from build123d import *

# Parameters (mm, degrees)
PAD_DEPTH       = 90
POCKET_DEPTH    = 8.9110010593
POCKET001_DEPTH = 7.0820946587


with BuildPart() as part:
    # Sketch → Pad (new body)
    with BuildSketch(Plane.YZ):
        with BuildLine():
            Line((-7, -25), (-4, -25))
            ThreePointArc((-4, -25), (-3.2928932188, -24.7071067812), (-3, -24))
            Line((-3, -24), (-3, 0))
            ThreePointArc((3, 0), (0, 1), (-3, 0))
            Line((3, 0), (3, -4))
            ThreePointArc((3, -4), (3.2928932188, -4.7071067812), (4, -5))
            Line((5.124826301, -5), (4, -5))
            ThreePointArc((5.124826301, -5), (5.6328573812, -4.8613387379), (6, -4.483808843))
            Line((14.00686173, 10), (6, -4.483808843))
            Line((14.00686173, 10), (14.00686173, 11.5))
            ThreePointArc((14.00686173, 11.5), (13.7139685112, 12.2071067812), (13.00686173, 12.5))
            Line((13.00686173, 12.5), (10.00686173, 12.5))
            ThreePointArc((10.00686173, 12.5), (9.2997549488, 12.2071067812), (9.00686173, 11.5))
            Line((9.00686173, 11.5), (9.00686173, 10))
            ThreePointArc((-2.99313827, 10), (3.00686173, 6.7888974491), (9.00686173, 10))
            Line((-2.99313827, 10), (-5.0865765197, 49.9451813902))
            ThreePointArc((-5.0865765197, 49.9451813902), (-5.4160754481, 50.6359902594), (-6.1375420107, 50.8914749687))
            Line((-6.1375420107, 50.8914749687), (-9.133430615, 50.7344671))
            ThreePointArc((-9.133430615, 50.7344671), (-9.8242394842, 50.4049681716), (-10.0797241935, 49.683501609))
            Line((-10.0797241935, 49.683501609), (-8, 10))
            Line((-8, 10), (-8, -24))
            ThreePointArc((-8, -24), (-7.7071067812, -24.7071067812), (-7, -25))
        make_face()
    extrude(amount=PAD_DEPTH)

    # Sketch002 (on Face1 of Pad) → Pocket (cut, through all)
    with BuildSketch(Plane(origin=(0, -2.4622975914, -0.1290435487), x_dir=(0, -0.0523359562, 0.9986295348), z_dir=(0, 0.9986295348, 0.0523359562))):
        with BuildLine():
            Line((51.1429441011, 75), (45.1429441011, 75))
            ThreePointArc((45.1429441011, 75), (15.1429441011, 45), (45.1429441011, 15))
            Line((45.1429441011, 15), (51.1429441011, 15))
            Line((51.1429441011, 15), (51.1429441011, 75))
        make_face()
    extrude(amount=-POCKET_DEPTH, mode=Mode.SUBTRACT)

    # Sketch003 (on Face17 of Pocket) → Pocket001 (cut, through all)
    with BuildSketch(Plane.ZX.offset(-3)):
        with BuildLine():
            Line((-75, 75), (-35, 75))
            ThreePointArc((-35, 15), (-5, 45), (-35, 75))
            Line((-35, 15), (-75, 15))
            Line((-75, 15), (-75, 75))
        make_face()
    extrude(amount=-POCKET001_DEPTH, mode=Mode.SUBTRACT)


solid = part.part
The listing builds one solid part. Answer for the finished solid, in the listing's coordinates (mm). A direction names the side the tool comes from. Round coordinates to 2 decimals unless told otherwise and drop trailing zeros. Order: outer loops, then holes, each group sorted by start corner. A loop starts at its lowest first (then second) coordinate and runs counter-clockwise, first axis right, second up. Notation, with made-up numbers: (73.5, -19) -> (106.5, -19) arc R14 ccw to (106.5, -8) -> close; hole circle Ø11 at (-18, -27). An arc over 180 degrees is marked (long way). Write each question's results on one line, items separated by ' | '. Start each with the question number.
Q1. Which of the six approach directions +Z, -Z, +X, -X, +Y, -Y give full straight-line access (tool end or side, diameter ignored) to faces 1 (the flat face through (44, 12, 12.5)), 2 (the flat face through (15, -7, 48)), 3 (the flat face through (44, -3, -4)), 4 (the flat face through (90, -3.4, 10.3))?
Q2. The mould has two halves that part along Y. Classify faces 5 (the flat face through (44, 3, -2)), 6 (the flat face through (44, -8, -3)), 7 (the flat face through (75, -7, 48)): pulls with the +Y half, pulls with the -Y half, needs draft (parallel to the pull), parting line crosses it, or undercut.
Q3. Find section A-A (x = 9). Determine the outline of the cut face in (y, z).
Q4. Find section D-D (x = 50). Determine the outline of the cut face in (y, z), then the cut area to 3 significant figures.
Q5. Find section B-B (z = -8). Determine the outline of the cut face in (x, y).
Q6. Find section C-C (y = 7.75). Determine the outline of the cut face in (x, z).
Q7. Each of these flat-tipped pins is pushed along its axis until it touches: pin 1 (1 mm diameter, centred on x = 68.5, y = 1, fed in from -Z); pin 2 (12 mm diameter, centred on x = 20.5, z = 7.5, fed in from -Y); pin 3 (1.2 mm diameter, centred on x = 43.5, z = 11, fed in from -Y). Where does it stop, or does it pass through?
Q8. Straight lines are drawn through the part: probe 1 along Y at (x, z) = (4.5, -18); probe 2 along Y at (x, z) = (36, -4.5); probe 3 along Y at (x, z) = (81, 47.5). For each, find the intervals that lie inside material, in ascending order. Write a range as from..to.
Worked answers:
1) face 1: +Z, +X, -X, +Y | face 2: +Z, +Y, -Y | face 3: -Z, +X, -X | face 4: +Z, -Z, +X, +Y, -Y
2) face 5: undercut | face 6: pulls with the -Y half | face 7: needs draft
3) outline: (-10.08, 49.68) -> (-8, 10) -> (-8, -24) arc R1 ccw to (-7, -25) -> (-4, -25) arc R1 ccw to (-3, -24) -> (-3, 0) arc R5 cw to (3, 0) -> (3, -4) arc R1 ccw to (4, -5) -> (5.12, -5) arc R1 ccw to (6, -4.48) -> (14.01, 10) -> (14.01, 11.5) arc R1 ccw to (13.01, 12.5) -> (10.01, 12.5) arc R1 ccw to (9.01, 11.5) -> (9.01, 10) arc R7.21 cw to (-2.99, 10) -> (-5.09, 49.95) arc R1 ccw to (-6.14, 50.89) -> (-9.13, 50.73) arc R1 ccw to start
4) outline: (-8.27, 15.15) -> (-8, 10) -> (-8, -5.42) -> (-3, -5.42) -> (-3, 0) arc R5 cw to (3, 0) -> (3, -4) arc R1 ccw to (4, -5) -> (5.12, -5) arc R1 ccw to (6, -4.48) -> (14.01, 10) -> (14.01, 11.5) arc R1 ccw to (13.01, 12.5) -> (10.01, 12.5) arc R1 ccw to (9.01, 11.5) -> (9.01, 10) arc R7.21 cw to (-2.99, 10) -> (-3.28, 15.41) -> close | area: 247 mm2
5) outline: (0, -8) -> (31.92, -8) -> (31.92, -3) -> (0, -3) -> close; (58.08, -8) -> (90, -8) -> (90, -3) -> (58.08, -3) -> close
6) outline: (0, -1.32) -> (90, -1.32) -> (90, 8.57) -> (0, 8.57) -> close
7) pin 1: stops at z = 0.77 | pin 2: stops at y = -8.18 | pin 3: stops at y = -8.08
8) probe 1: y = -8..-3 | probe 2: y = -8..-3, 3.13..5.99 | probe 3: y = -9.97..-4.96
